Design review of the part built by this model. Coordinates are the model's own, in mm. A direction names the side the tool comes from. Give positions to 0.01 mm unless a question says otherwise; leave off trailing zeros. Order: outer loops, then holes, each group sorted by start corner. A loop starts at its lowest first (then second) coordinate and runs counter-clockwise, first axis right, second up. Notation, with made-up numbers: (12.25, -37.75) -> (59.25, -37.75) arc R27 cw to (59.25, -3.75) -> close; hole circle Ø1 at (9, -23.75). An arc over 180 degrees is marked (long way). Return JSON: item names as keys, results as strings.
```python
from build123d import *

# Parameters (mm, degrees)
SKETCH1_W           = 72
SKETCH1_H           = 72
BOSS_EXTRUDE1_DEPTH = 40
SKETCH3_W           = 60
SKETCH3_H           = 60
CUT_EXTRUDE1_DEPTH  = 10
SKETCH4_R           = 2.5
CUT_EXTRUDE2_DEPTH  = 30
SKETCH5_R           = 19.075
CUT_EXTRUDE3_DEPTH  = 27
CUT_EXTRUDE5_DEPTH  = 27
SKETCH13_R          = 3
BOSS_EXTRUDE3_DEPTH = 10


with BuildPart() as part:
    # Sketch1 → Boss-Extrude1 (new body)
    with BuildSketch(Plane(origin=(0, 0, 0), x_dir=(1, 0, 0), z_dir=(0, 1, 0))):
        Rectangle(SKETCH1_W, SKETCH1_H)
    extrude(amount=BOSS_EXTRUDE1_DEPTH)

    # Sketch3 → Cut-Extrude1 (cut)
    with BuildSketch(Plane(origin=(0, 40, 0), x_dir=(1, 0, 0), z_dir=(0, 1, 0))):
        Rectangle(SKETCH3_W, SKETCH3_H)
    extrude(amount=-CUT_EXTRUDE1_DEPTH, mode=Mode.SUBTRACT)

    # Sketch4 → Cut-Extrude2 (cut)
    with BuildSketch(Plane(origin=(0, 30, 0), x_dir=(1, 0, 0), z_dir=(0, 1, 0))):
        with Locations((-23.57, 23.57)):
            Circle(SKETCH4_R)
        with Locations((23.57, 23.57)):
            Circle(SKETCH4_R)
        with Locations((23.57, -23.57)):
            Circle(SKETCH4_R)
        with Locations((-23.57, -23.57)):
            Circle(SKETCH4_R)
    extrude(amount=-CUT_EXTRUDE2_DEPTH, mode=Mode.SUBTRACT)

    # Sketch5 → Cut-Extrude3 (cut)
    with BuildSketch(Plane(origin=(0, 30, 0), x_dir=(1, 0, 0), z_dir=(0, 1, 0))):
        Circle(SKETCH5_R)
    extrude(amount=-CUT_EXTRUDE3_DEPTH, mode=Mode.SUBTRACT)

    # Sketch6 → Cut-Extrude5 (cut)
    with BuildSketch(Plane(origin=(0, 30, 0), x_dir=(1, 0, 0), z_dir=(0, 1, 0))):
        with BuildLine():
            Line((-13.99552044, 12.960749693), (-18.030218489, 36))
            Line((-18.030218489, 36), (18.058704295, 36))
            Line((18.058704295, 36), (13.99552044, 12.960749693))
            ThreePointArc((13.99552044, 12.960749693), (0, 19.075), (-13.99552044, 12.960749693))
        make_face()
    extrude(amount=-CUT_EXTRUDE5_DEPTH, mode=Mode.SUBTRACT)

    # Sketch13 → Boss-Extrude3 (add)
    with BuildSketch(Plane.XZ):
        with Locations((0, 23.57)):
            Circle(SKETCH13_R)
        with Locations((23.57, 0)):
            Circle(SKETCH13_R)
        with Locations((-23.57, 0)):
            Circle(SKETCH13_R)
    extrude(amount=BOSS_EXTRUDE3_DEPTH)


solid = part.part
```
Item 1: Add section A-A (z = 23.57). Give the boundary of the cut face in (x, y), plus the area to 3 significant figures.
Result set:
{"outline": "(-36, 0) -> (-26.07, 0) -> (-26.07, 30) -> (-30, 30) -> (-30, 40) -> (-36, 40) -> close; (-21.07, 0) -> (-3, 0) -> (-3, -10) -> (3, -10) -> (3, 0) -> (21.07, 0) -> (21.07, 30) -> (-21.07, 30) -> close; (26.07, 0) -> (36, 0) -> (36, 40) -> (30, 40) -> (30, 30) -> (26.07, 30) -> close", "area": "2,040 mm^2"}
Item 2: Add section B-B (x = 0). Give the boundary of the cut face in (y, z) (3 decimals), plus the area to 3 significant figures.
Result set:
{"outline": "(-10, 20.57) -> (0, 20.57) -> (0, -36) -> (3, -36) -> (3, 19.075) -> (30, 19.075) -> (30, 30) -> (40, 30) -> (40, 36) -> (0, 36) -> (0, 26.57) -> (-10, 26.57) -> close; (30, -36) -> (40, -36) -> (40, -30) -> (30, -30) -> close", "area": "853 mm^2"}
Item 3: Wall thickness on L1, parallel to Z at x = -23.57, y = 14.25; L2, parallel to Z at x = 6, y = 36; L3, parallel to X at y = 14, z = 23: over which ranges is each line inside the solid? List them lowest first. Write a range as [from, to].
Result set:
{"L1": "z = [-36, -26.07], [-21.07, 21.07], [26.07, 36]", "L2": "z = [-36, -30], [30, 36]", "L3": "x = [-36, -26], [-21.14, 21.14], [26, 36]"}
Item 4: Machinability: for faces 4 (the face through (0, 35, 30)), 5 (the face through (16.056, 16.689, -24.642)), 6 (the face through (-20.8, -4.93, -1.15)), which of the approach directions +Z, -Z, +X, -X, +Y, -Y give a long, thin tool a straight path to every point of the face, cutting with its end or side? Answer none if there is none.
Result set:
{"face 4": "+Y", "face 5": "-Z", "face 6": "-Y"}
Item 5: Add section D-D (x = 23.57). Give the boundary of the cut face in (y, z).
Result set:
{"outline": "(-10, -3) -> (0, -3) -> (0, -21.07) -> (30, -21.07) -> (30, 21.07) -> (0, 21.07) -> (0, 3) -> (-10, 3) -> close; (0, -36) -> (40, -36) -> (40, -30) -> (30, -30) -> (30, -26.07) -> (0, -26.07) -> close; (0, 26.07) -> (30, 26.07) -> (30, 30) -> (40, 30) -> (40, 36) -> (0, 36) -> close"}
Item 6: For pin 1 (6 mm diameter, centred on x = 16, z = 15.5, fed in from -Y); pin 2 (3 mm diameter, centred on x = 23.57, z = -23.57, fed in from -Y); pin 3 (6 mm diameter, centred on x = -23.57, z = -23.57, fed in from +Y); pin 4 (4 mm diameter, centred on x = 14.5, z = -3.5, fed in from +Y), all flat-tipped, find the tip position at first contact; note any pin that passes through.
Result set:
{"pin 1": "stops at y = 0", "pin 2": "passes through", "pin 3": "stops at y = 30", "pin 4": "stops at y = 3"}
Item 7: Mouldability with a two-part tool opening along Y and no side actions: class faces 1 (the face through (0, -10, 24)), 2 (the face through (-15.985, 16.689, -24.319)), 3 (the face through (20.573, -4.93, 0.132)) as released by +Y, released by -Y, zero draft, split by the parting line, or undercut.
Result set:
{"face 1": "released by -Y", "face 2": "undercut", "face 3": "zero draft"}
Item 8: Add section C-C (y = 12). Give the boundary of the cut face in (x, z) (3 decimals), plus the area to 3 significant figures.
Result set:
{"outline": "(-36, -36) -> (-18.03, -36) -> (-13.996, -12.961) arc R19.075 cw (long way) to (13.996, -12.961) -> (18.059, -36) -> (36, -36) -> (36, 36) -> (-36, 36) -> close; hole circle Ø5 at (-23.57, -23.57); hole circle Ø5 at (-23.57, 23.57); hole circle Ø5 at (23.57, -23.57); hole circle Ø5 at (23.57, 23.57)", "area": "3,340 mm^2"}
